Could you check a few things on this model? Use its own coordinates, in mm. Give positions to 0.01 mm unless a question says otherwise; leave off trailing zeros. Loops run counter-clockwise (first coordinate to the right, second up) from the corner with the lowest first, then second, coordinate; pieces in that order, holes last. Notation, with made-up numbers: (57, 41) - (68, 41) arc R21 cw to (68, 59) - close; hole circle Ø3 at (28, 32.5). An arc over 180 degrees is marked (long way). One line per item, written item: value. Start each with the question number.
Q1. I want a section at D-D (y = 23.5). Please give me the cut outline in (x, z), then the cut area to 3 significant figures.
Q2. I want a section at A-A (x = -25). Please give me the cut outline in (y, z).
Q3. I'm going to push flat-ended pins straight in: P1, Ø2, axis at x = -13.5, z = 8, coming from the -Y side; P2, Ø8, axis at x = 44.38, y = 76.87, coming from the -Z side; P3, Ø5, axis at y = 250, z = 3, coming from the +X side; P4, Ø1.5, axis at x = 154, z = 5, coming from the +Y side. Where does each tip first touch, or does it pass through?
Q4. I want a section at C-C (z = 5.75). Please give me the cut outline in (x, y).
Q5. If I drill on line 1 (X direction, y = 134, z = 5.25); line 2 (X direction, y = 223, z = 3); line 3 (X direction, y = 259, z = 2.25), over which ranges is the centre line in solid material (lowest first)? Write a range as from..to.
Q6. I want a section at B-B (y = 119). Please give me the cut outline in (x, z), then the cut area to 3 significant figures.
```python
from build123d import *

# Parameters (mm, degrees)
F0_R     = 5
F1_DEPTH = 9.5


with BuildPart() as f1:
    # F0 (on Top) → F1 (new body)
    with BuildSketch(Plane.XY):
        with BuildLine():
            ThreePointArc((27.091291, 212.009885), (24.224301, 218.341531), (17.923315, 221.275292))
            ThreePointArc((17.923315, 221.275292), (8.96898, 221.818749), (0, 222))
            Line((0, 222), (0, 272))
            ThreePointArc((0, 272), (-25.10719, 270.838751), (-50, 267.364919))
            Line((-50, 267.364919), (-50, 73.627441))
            Line((-50, 73.627441), (88.763234, -6.48755))
            Line((88.763234, -6.48755), (256.544812, 90.381189))
            ThreePointArc((256.544812, 90.381189), (247.106834, 113.675911), (235.55891, 136))
            Line((235.55891, 136), (192.25764, 111))
            ThreePointArc((192.25764, 111), (187.616182, 118.676739), (182.668367, 126.159692))
            ThreePointArc((182.668367, 126.159692), (176.977162, 130.149626), (170.0603, 129.466689))
            Line((170.0603, 129.466689), (110.29109, 100.347803))
            ThreePointArc((110.29109, 100.347803), (101.586655, 98.98529), (93.61871, 102.745011))
            ThreePointArc((93.61871, 102.745011), (69.5, 120.377531), (42.170434, 132.448686))
            ThreePointArc((42.170434, 132.448686), (34.930449, 137.469269), (31.758201, 145.688787))
            Line((31.758201, 145.688787), (27.091291, 212.009885))
        make_face()
        with Locations((44.382053, 76.870964)):
            Circle(F0_R, mode=Mode.SUBTRACT)
        with Locations((205.15145, 89.576731)):
            Circle(F0_R, mode=Mode.SUBTRACT)
        with Locations((-25, 222)):
            Circle(F0_R, mode=Mode.SUBTRACT)
    extrude(amount=F1_DEPTH)


solid = f1.part
```
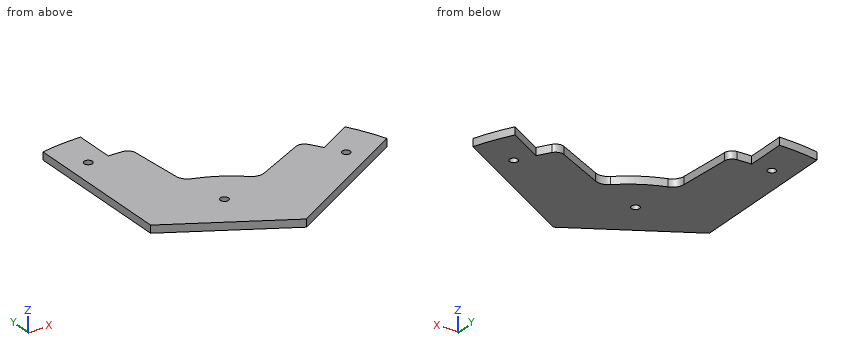
Worked answers:
1. outline: (36.82, 0) - (140.7, 0) - (140.7, 9.5) - (36.82, 9.5) - close
1. area: 987 mm²
2. outline: (59.19, 0) - (217, 0) - (217, 9.5) - (59.19, 9.5) - close; (227, 0) - (270.85, 0) - (270.85, 9.5) - (227, 9.5) - close
3. P1: stops at y = 51.98
3. P2: passes through
3. P3: stops at x = 0
3. P4: stops at y = 122.01
4. outline: (-50, 73.63) - (88.76, -6.49) - (256.54, 90.38) arc R272 ccw to (235.56, 136) - (192.26, 111) arc R222 ccw to (182.67, 126.16) arc R10 ccw to (170.06, 129.47) - (110.29, 100.35) arc R15 cw to (93.62, 102.75) arc R139 ccw to (42.17, 132.45) arc R15 cw to (31.76, 145.69) - (27.09, 212.01) arc R10 ccw to (17.92, 221.28) arc R222 ccw to (0, 222) - (0, 272) arc R272 ccw to (-50, 267.36) - close; hole circle Ø10 at (-25, 222); hole circle Ø10 at (44.38, 76.87); hole circle Ø10 at (205.15, 89.58)
5. line 1: x = -50..38.81, 232.09..236.7
5. line 2: x = -50..-29.9, -20.1..0
5. line 3: x = -50..0
6. outline: (-50, 0) - (71.83, 0) - (71.83, 9.5) - (-50, 9.5) - close; (148.58, 0) - (187.41, 0) - (187.41, 9.5) - (148.58, 9.5) - close; (206.11, 0) - (244.59, 0) - (244.59, 9.5) - (206.11, 9.5) - close
6. area: 1,890 mm²
